Design review of the part built by this model. Coordinates are the model's own, in mm. A direction names the side the tool comes from. Coordinates: 2 decimals unless noted, no trailing zeros. Write each loop counter-clockwise with the first axis right and the second up, starting at its lowest first coordinate (ties: lowest second). Pieces come first, ordered by that corner, then holes. Notation, with made-up numbers: (29.25, -35) - (76.25, -35) arc R16 ccw to (76.25, -26) - close; hole circle Ø11 at (69, -2). An arc over 180 degrees is marked (long way). Use a Markdown table: item, result.
from build123d import *

# Parameters (mm, degrees)
F1_DEPTH  = 6.35
F2_R      = 3.175
F3_W      = 76.2
F3_H      = 2.54
F4_DEPTH  = 10.16
F5_SIZE   = 5.08
F7_DEPTH  = 6.35
F8_SIZE   = 5.08
F10_D     = 2.2606
F13_DEPTH = 5.08
F14_R     = 5.3951847675
F15_REACH = 89.7970127444
F17_D     = 3.4544
F19_D     = 6.35
F19_DEPTH = 2.541


with BuildPart() as f1:
    # F0 (on Front) → F1 (new body)
    with BuildSketch(Plane.XZ):
        Polygon((9.525, 88.9), (-9.525, 88.9), (-53.7482142857, 6.35), (-57.15, 0), (57.15, 0), (53.7482142857, 6.35), align=None)
        with BuildLine():
            Line((41.2416306314, 6.35), (-41.2416306314, 6.35))
            ThreePointArc((-41.2416306314, 6.35), (-43.9656820238, 7.8939975439), (-44.0403295363, 11.0243029847))
            Line((-44.0403295363, 11.0243029847), (-35.876043822, 26.2643029847))
            ThreePointArc((-35.876043822, 26.2643029847), (-34.7083473732, 27.4890513924), (-33.0773449171, 27.94))
            Line((-33.0773449171, 27.94), (33.0773449171, 27.94))
            ThreePointArc((33.0773449171, 27.94), (34.7083473732, 27.4890513924), (35.876043822, 26.2643029847))
            Line((35.876043822, 26.2643029847), (44.0403295363, 11.0243029847))
            ThreePointArc((44.0403295363, 11.0243029847), (43.9656820238, 7.8939975439), (41.2416306314, 6.35))
        make_face(mode=Mode.SUBTRACT)
        with BuildLine():
            ThreePointArc((-14.1046152506, 66.9043029847), (-12.9369188018, 68.1290513924), (-11.3059163457, 68.58))
            Line((-11.3059163457, 68.58), (11.3059163457, 68.58))
            ThreePointArc((11.3059163457, 68.58), (12.9369188018, 68.1290513924), (14.1046152506, 66.9043029847))
            Line((14.1046152506, 66.9043029847), (29.0724723934, 38.9643029847))
            ThreePointArc((29.0724723934, 38.9643029847), (28.9978248809, 35.8339975439), (26.2737734886, 34.29))
            Line((26.2737734886, 34.29), (-26.2737734886, 34.29))
            ThreePointArc((-26.2737734886, 34.29), (-28.9978248809, 35.8339975439), (-29.0724723934, 38.9643029847))
            Line((-29.0724723934, 38.9643029847), (-14.1046152506, 66.9043029847))
        make_face(mode=Mode.SUBTRACT)
        Polygon((-57.15, 0), (-53.7482142857, 6.35), (-57.15, 6.35), align=None)
        Polygon((57.15, 6.35), (53.7482142857, 6.35), (57.15, 0), align=None)
    extrude(amount=F1_DEPTH)

    # F2
    f2_edges = [f1.edges().sort_by_distance(p)[0] for p in [
        (53.748214, -3.175, 6.35),
        (-53.748214, -3.175, 6.35),
    ]]
    fillet(f2_edges, radius=F2_R)

    # F3 (on face) → F4 (join)
    with BuildSketch(Plane.XZ.offset(6.35)):
        with Locations((0, 1.27)):
            Rectangle(F3_W, F3_H)
    extrude(amount=F4_DEPTH)

    # F5
    f5_edges = [f1.edges().sort_by_distance(p)[0] for p in [
        (-38.1, -16.51, 1.27),
        (38.1, -16.51, 1.27),
    ]]
    chamfer(f5_edges, length=F5_SIZE)

    # F6 (on face) → F7 (join)
    with BuildSketch(Plane.XZ.offset(6.35)):
        Polygon((-42.1821428571, 27.94), (-33.0773449171, 27.94), (-26.4341428571, 27.94), (-26.4341428571, 34.29), (-38.7803571429, 34.29), align=None)
        Polygon((26.4341428571, 34.29), (26.4341428571, 27.94), (33.0773449171, 27.94), (42.1821428571, 27.94), (38.7803571429, 34.29), align=None)
    extrude(amount=F7_DEPTH)

    # F8
    f8_edges = [f1.edges().sort_by_distance(p)[0] for p in [
        (26.434143, -12.7, 31.115),
        (-26.434143, -12.7, 31.115),
    ]]
    chamfer(f8_edges, length=F8_SIZE)

    # F10 (through all)
    with Locations(Plane.XZ.offset(12.7)):
        with Locations((-34.163, 31.242), (34.163, 31.242)):
            Hole(F10_D / 2)



with BuildPart() as f13:
    # F12 (on face) → F13 (new body)
    with BuildSketch(Plane(origin=(0, 44.45, 44.45), x_dir=(-1, 0, 0), z_dir=(0, 0.7071067812, 0.7071067812))):
        Polygon((-3.6661742094, 48.8917928475), (3.6661742094, 48.8917928475), (7.3323484187, 55.2417928475), (3.6661742094, 61.5917928475), (-3.6661742094, 61.5917928475), (-7.3323484187, 55.2417928475), align=None)
    extrude(amount=F13_DEPTH)


with BuildPart() as f1_1:
    add(f1.part)

    add(f13.part)  # F15 merges F13
    f15_end = f1_1.faces().sort_by_distance((-29.9113566426, 0, 47.7790611404))[0]
    # F14 (on face) → F15 (join, up to a face of the model that its end follows)
    with BuildSketch(Plane(origin=(0, 44.45, 44.45), x_dir=(1, 0, 0), z_dir=(0, -0.7071067812, -0.7071067812))):
        with Locations((0, 55.2417928475)):
            Circle(F14_R)
    f15_long = extrude(amount=F15_REACH, mode=Mode.PRIVATE)
    add(split(f15_long, bisect_by=f15_end, keep=Keep.TOP, mode=Mode.PRIVATE))

    # F17 (through all)
    with Locations(Plane(origin=(0, 48.0421024484, 48.0421024484), x_dir=(-1, 0, 0), z_dir=(0, 0.7071067812, 0.7071067812))):
        with Locations((0, 55.2417928475)):
            Hole(F17_D / 2)

    # F19 (through all, one way)
    with BuildSketch(Plane.XY.offset(2.54)):
        with Locations((-25.4, -9.525), (25.4, -9.525)):
            Circle(F19_D / 2)
    extrude(amount=-F19_DEPTH, mode=Mode.SUBTRACT)


solid = f1_1.part
(1) For pin 1 (10 mm diameter, centred on y = -10, z = 38.5, fed in from +X); pin 2 (1.2 mm diameter, centred on x = 56.5, y = -3, fed in from +Z); pin 3 (3 mm diameter, centred on x = -1.5, y = -9.5, fed in from +Z); pin 4 (10 mm diameter, centred on x = 28, z = 75, fed in from -Y), all flat-tipped, find the tip position at first contact; note any pin that passes through.
Determined:
| item | result |
|---|---|
| pin 1 | x = 39.2 |
| pin 2 | z = 6.35 |
| pin 3 | z = 2.54 |
| pin 4 | through |
(2) Take a section at C-C on y = -2.75. State how many separate pieces and enclosed holes the cut face has, and give its area (3 significant figures).
Determined:
| item | result |
|---|---|
| separate pieces | 1 |
| enclosed holes | 5 |
| area | 2,660 mm2 |
(3) Take a section at B-B on x = -40. Write out the cut boundary in (y, z).
Determined:
| item | result |
|---|---|
| outline | (-12.7, 27.94) - (-6.35, 27.94) - (-6.35, 18.57) - (0, 18.57) - (0, 32.01) - (-12.7, 32.01) - close; (-6.35, 0) - (0, 0) - (0, 6.35) - (-6.35, 6.35) - close |
(4) Take a section at A-A on z = 48. Write out the cut boundary in (x, y), and give its area (3 significant figures).
Determined:
| item | result |
|---|---|
| outline | (-31.44, -6.35) - (-24.23, -6.35) - (-24.23, 0) - (-31.44, 0) - close; (24.23, -6.35) - (31.44, -6.35) - (31.44, 0) - (24.23, 0) - close |
| area | 91.5 mm2 |
(5) Machinability: for faces 5 (the flat face through (-5.525, 4.945, 87.496)), 6 (the flat face through (34, -9, 34.29)), 7 (the cylindrical face through (43.989, -3.131, 7.933)), which of the approach directions +Z, -Z, +X, -X, +Y, -Y give a long, thin tool a straight path to every point of the face, cutting with its end or side? Answer none if there is none.
Determined:
| item | result |
|---|---|
| face 5 | +Z, -X |
| face 6 | +Z, +X, -X, -Y |
| face 7 | +Y, -Y |
(6) For L1, parallel to Z at x = 8, y = -4.75; L2, parallel to Z at x = 36.5, y = -11.5; L3, parallel to X at y = -10, z = 32, list the stretches that pass through material, from the lowest coordinate up. Write a range as from..to.
Determined:
| item | result |
|---|---|
| L1 | 0..6.35, 27.94..34.29, 68.58..88.9 |
| L2 | 0..2.54, 27.94..34.29 |
| L3 | -40.01..-35, -33.32..-28.81, 28.81..33.32, 35..40.01 |
(7) Draft analysis for pull direction X (two halves, no side actions). For faces 1 (the flat face through (5.525, 9.373, 83.069)), 2 (the cylindrical face through (29.02, -3.13, 35.87)), 3 (the flat face through (-5.474, 9.436, 83.006)), 4 (the flat face through (-1, -11, 2.54)), state which applies: +X half, -X half, draft (parallel to the pull), parting line (faces both ways), or undercut.
Determined:
| item | result |
|---|---|
| face 1 | +X half |
| face 2 | undercut |
| face 3 | -X half |
| face 4 | draft |
